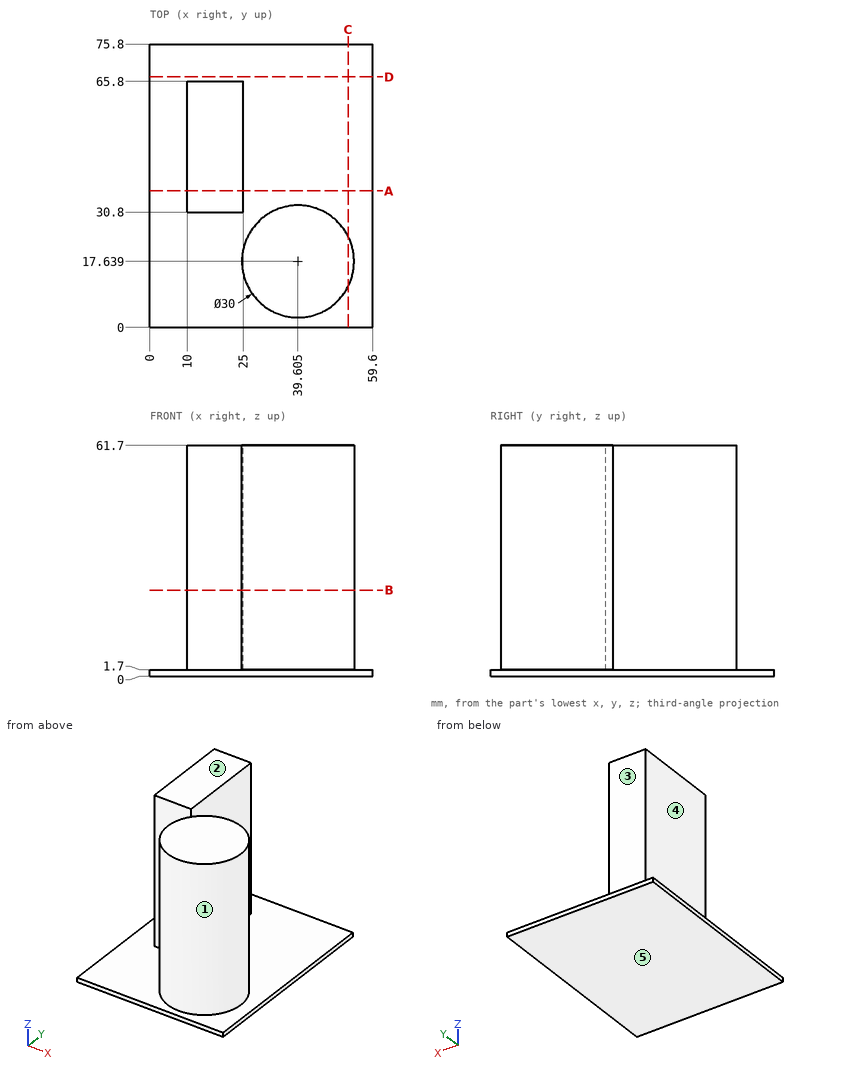
Drawing for the job (mm, zero at the part's lowest x, y, z). A direction names the side the tool comes from. Coordinates: 2 decimals unless noted, no trailing zeros. Write each loop counter-clockwise with the first axis right and the second up, starting at its lowest first coordinate (ties: lowest second). Pieces come first, ordered by that corner, then holes. Notation, with made-up numbers: (66.5, 40.5) -> (110.5, 40.5) arc R23 ccw to (110.5, 71.5) -> close; hole circle Ø1 at (64.25, 34). An arc over 180 degrees is marked (long way). One line per item, written item: value. Start each with the question number.
1) Flat gauge pins, fed straight in: pin 1 Ø12 at (x, z) = (27.5, 47.5) entering from +Y; pin 2 Ø5 at (x, y) = (52.5, 30.5) entering from +Z; pin 3 Ø1 at (x, z) = (48, 14) entering from -Y (1 decimal). Where does each tip first touch, or does it go through?
2) Probe probe 1 along Z at (x, y) = (18.5, 24); probe 2 along Y at (x, z) = (39, 51.5); probe 3 along Y at (x, z) = (15, 14). List the from-to ranges inside material, lowest first.
3) Slice it at A-A on y = 36.5. Write the cut outline in (x, z), then the cut area to 3 significant figures.
4) Slice it at B-B on z = 23. Write the cut outline in (x, y) (1 decimal), then the cut area to 3 significant figures.
5) Slice it at C-C on x = 53. Write the cut outline in (y, z), then the cut area to 3 significant figures.
6) Slice it at D-D on y = 67. Write the cut outline in (x, z), then the cut area to 3 significant figures.
7) Which spindle directions (+Z, -Z, +X, -X, +Y, -Y) get a long thin tool onto all of the face, cutting with end or side? Do the marked faces 1, 2, 3, 4 and 5. Say none if no direction does.
Answers follow:
1. pin 1: y = 65.8
1. pin 2: z = 1.7
1. pin 3: y = 4.9
2. probe 1: 0 to 1.7
2. probe 2: 2.65 to 32.63
2. probe 3: 30.8 to 65.8
3. outline: (0, 0) -> (59.6, 0) -> (59.6, 1.7) -> (25, 1.7) -> (25, 61.7) -> (10, 61.7) -> (10, 1.7) -> (0, 1.7) -> close
3. area: 1,000 mm2
4. outline: (10, 30.8) -> (25, 30.8) -> (25, 65.8) -> (10, 65.8) -> close; circle Ø30 at (39.6, 17.6)
4. area: 1,230 mm2
5. outline: (0, 0) -> (75.8, 0) -> (75.8, 1.7) -> (24.39, 1.7) -> (24.39, 61.7) -> (10.89, 61.7) -> (10.89, 1.7) -> (0, 1.7) -> close
5. area: 939 mm2
6. outline: (0, 0) -> (59.6, 0) -> (59.6, 1.7) -> (0, 1.7) -> close
6. area: 101 mm2
7. face 1: +Z
7. face 2: +Z, +X, -X, +Y, -Y
7. face 3: +Z, +X, -X, +Y
7. face 4: +Z, -X, +Y, -Y
7. face 5: -Z, +X, -X, +Y, -Y
